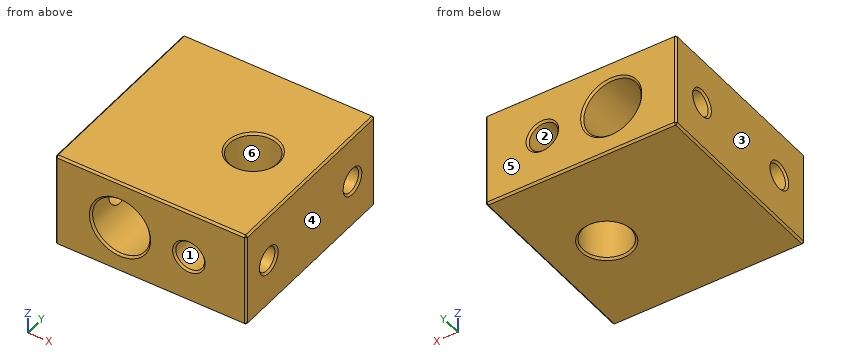
from build123d import *

# Parameters (mm, degrees)
SKETCH_1_W          = 20
SKETCH_1_H          = 20
EXTRUDE_1_DEPTH     = 10
SKETCH_2_R          = 2.5
CUT_EXTRUDE_1_DEPTH = 10
SKETCH_3_R          = 3
CUT_EXTRUDE_2_DEPTH = 20
SKETCH_4_R          = 1.25
CUT_EXTRUDE_3_DEPTH = 6.7
SKETCH_5_R          = 1.5
CUT_EXTRUDE_4_DEPTH = 6
SKETCH_6_R          = 1.5
CUT_EXTRUDE_5_DEPTH = 6
SKETCH_7_R          = 1.25
CUT_EXTRUDE_6_DEPTH = 6
CHAMFER_1_SIZE      = 0.2


with BuildPart() as part:
    # Эскиз1 → Бобышка-Вытянуть1 (new body)
    with BuildSketch(Plane.XY):
        with Locations((10, 10)):
            Rectangle(SKETCH_1_W, SKETCH_1_H)
    extrude(amount=EXTRUDE_1_DEPTH)

    # Эскиз2 → Вырез-Вытянуть1 (cut)
    with BuildSketch(Plane.XY.offset(10)):
        with Locations((14, 10)):
            Circle(SKETCH_2_R)
    extrude(amount=-CUT_EXTRUDE_1_DEPTH, mode=Mode.SUBTRACT)

    # Эскиз3 → Вырез-Вытянуть2 (cut)
    with BuildSketch(Plane.XZ):
        with Locations((6.8, 5)):
            Circle(SKETCH_3_R)
    extrude(amount=-CUT_EXTRUDE_2_DEPTH, mode=Mode.SUBTRACT)

    # Эскиз4 → Вырез-Вытянуть3 (cut)
    with BuildSketch(Plane.ZY):
        with Locations((5, 16)):
            Circle(SKETCH_4_R)
        with Locations((5, 4)):
            Circle(SKETCH_4_R)
    extrude(amount=-CUT_EXTRUDE_3_DEPTH, mode=Mode.SUBTRACT)

    # Эскиз5 → Вырез-Вытянуть4 (cut)
    with BuildSketch(Plane.XZ):
        with Locations((14, 5)):
            Circle(SKETCH_5_R)
    extrude(amount=-CUT_EXTRUDE_4_DEPTH, mode=Mode.SUBTRACT)

    # Эскиз6 → Вырез-Вытянуть5 (cut)
    with BuildSketch(Plane(origin=(0, 20, 0), x_dir=(1, 0, 0), z_dir=(0, 1, 0))):
        with Locations((14, -5)):
            Circle(SKETCH_6_R)
    extrude(amount=-CUT_EXTRUDE_5_DEPTH, mode=Mode.SUBTRACT)

    # Эскиз7 → Вырез-Вытянуть6 (cut)
    with BuildSketch(Plane(origin=(20, 0, 0), x_dir=(0, 0, -1), z_dir=(1, 0, 0))):
        with Locations((-5, 3.5)):
            Circle(SKETCH_7_R)
        with Locations((-5, 16.5)):
            Circle(SKETCH_7_R)
    extrude(amount=-CUT_EXTRUDE_6_DEPTH, mode=Mode.SUBTRACT)

    # Фаска1
    chamfer_1_edges = [part.edges().sort_by_distance(p)[0] for p in [
        (20, 10, 10),
        (10, 20, 10),
        (11.5, 10, 0),
        (11.5, 10, 10),
        (3.8, 20, 5),
        (3.8, 0, 5),
        (0, 16, 3.75),
        (0, 4, 3.75),
        (12.5, 0, 5),
        (12.5, 20, 5),
        (0, 10, 10),
        (20, 3.5, 6.25),
        (10, 20, 0),
        (20, 10, 0),
        (20, 16.5, 6.25),
        (10, 0, 0),
        (0, 10, 0),
        (10, 0, 10),
        (0, 20, 5),
        (20, 20, 5),
        (20, 0, 5),
        (0, 0, 5),
    ]]
    chamfer(chamfer_1_edges, length=CHAMFER_1_SIZE)


solid = part.part
Build history of the part. All positions in model axes, mm. Face numbers are marked on the shaded views. A direction names the side the tool comes from. Round coordinates to 2 decimals unless told otherwise and drop trailing zeros. Write each loop counter-clockwise with the first axis right and the second up, starting at its lowest first coordinate (ties: lowest second). Pieces come first, ordered by that corner, then holes. Notation, with made-up numbers: M 8,56.5 L 53,56.5 A30 cw 53,88.5 Z; hole C -17,78.25 d9. An arc over 180 degrees is marked long. Answer as a JSON object with one key per item and string values. Group by question number.
(1) Cut at A-A (y = 10). Give the cut face in (x, z), and give its area (3 significant figures).
(2) Which spindle directions (+Z, -Z, +X, -X, +Y, -Y) get a long thin tool onto all of the face, cutting with end or side? Do the marked faces 1, 2 and 3. Say none if no direction does.
(3) Cut at C-C (z = 9.25). Give the cut face in (x, y), and give its area (3 significant figures).
(4) Cut at B-B (x = 6.8). Give the cut face in (y, z), and give its area (3 significant figures).
(5) Cut at D-D (z = 5). Give the number of separate pieces and of enclosed holes in the cut face, and give its area (3 significant figures).
(6) Drill centre lines: L1, parallel to Y at x = 1.4, z = 5; L2, parallel to Z at x = 18.6, y = 3.5; L3, parallel to Z at x = 6.8, y = 4.5. Where is each one in solid material? Low to high.
(7) Mould opens along Y. For the marked faces 4, 5 and 6 say: pulls with the +Y half, pulls with the -Y half, needs draft (parallel to the pull), parting line crosses it, or undercut.
(8) Flat gauge pins, fed straight in: pin 1 (1.5 mm diameter, centred on x = 14, z = 5.5, fed in from -Y); pin 2 (2 mm diameter, centred on y = 3.5, z = 5, fed in from +X); pin 3 (0.9 mm diameter, centred on x = 14, z = 4.5, fed in from +Y); pin 4 (4 mm diameter, centred on x = 14, y = 10, fed in from -Z). Where does each tip first touch, or does it go through?
Responses:
{
 "1": {"outline": "M 0,0.2 L 0.2,0 L 11.3,0 L 11.5,0.2 L 11.5,9.8 L 11.3,10 L 0.2,10 L 0,9.8 Z; M 16.5,0.2 L 16.7,0 L 19.8,0 L 20,0.2 L 20,9.8 L 19.8,10 L 16.7,10 L 16.5,9.8 Z; hole C 6.8,5 d6", "area": "122 mm2"},
 "2": {"face 1": "-Y", "face 2": "+Y", "face 3": "+Z, -Z, -X, +Y, -Y"},
 "3": {"outline": "M 0,0.2 L 0.2,0 L 19.8,0 L 20,0.2 L 20,19.8 L 19.8,20 L 0.2,20 L 0,19.8 Z; hole C 14,10 d5", "area": "380 mm2"},
 "4": {"outline": "M 0,0.2 L 0.2,0 L 19.8,0 L 20,0.2 L 20,1.8 L 19.8,2 L 0.2,2 L 0,1.8 Z; M 0,8.2 L 0.2,8 L 19.8,8 L 20,8.2 L 20,9.8 L 19.8,10 L 0.2,10 L 0,9.8 Z", "area": "79.8 mm2"},
 "5": {"separate pieces": "6", "enclosed holes": "1", "area": "182 mm2"},
 "6": {"L1": "y = 0 to 2.75, 5.25 to 14.75, 17.25 to 20", "L2": "z = 0 to 3.75, 6.25 to 10", "L3": "z = 0 to 2, 8 to 10"},
 "7": {"face 4": "needs draft", "face 5": "pulls with the +Y half", "face 6": "undercut"},
 "8": {"pin 1": "stops at y = 6", "pin 2": "stops at x = 12.88", "pin 3": "stops at y = 14", "pin 4": "passes through"}
}
